Geometry check sheet. Reference: drawing and pictorial views, mm from the part's lowest x, y, z. A direction names the side the tool comes from. Give positions to 0.01 mm unless a question says otherwise; leave off trailing zeros. Order: outer loops, then holes, each group sorted by start corner. A loop starts at its lowest first (then second) coordinate and runs counter-clockwise, first axis right, second up.
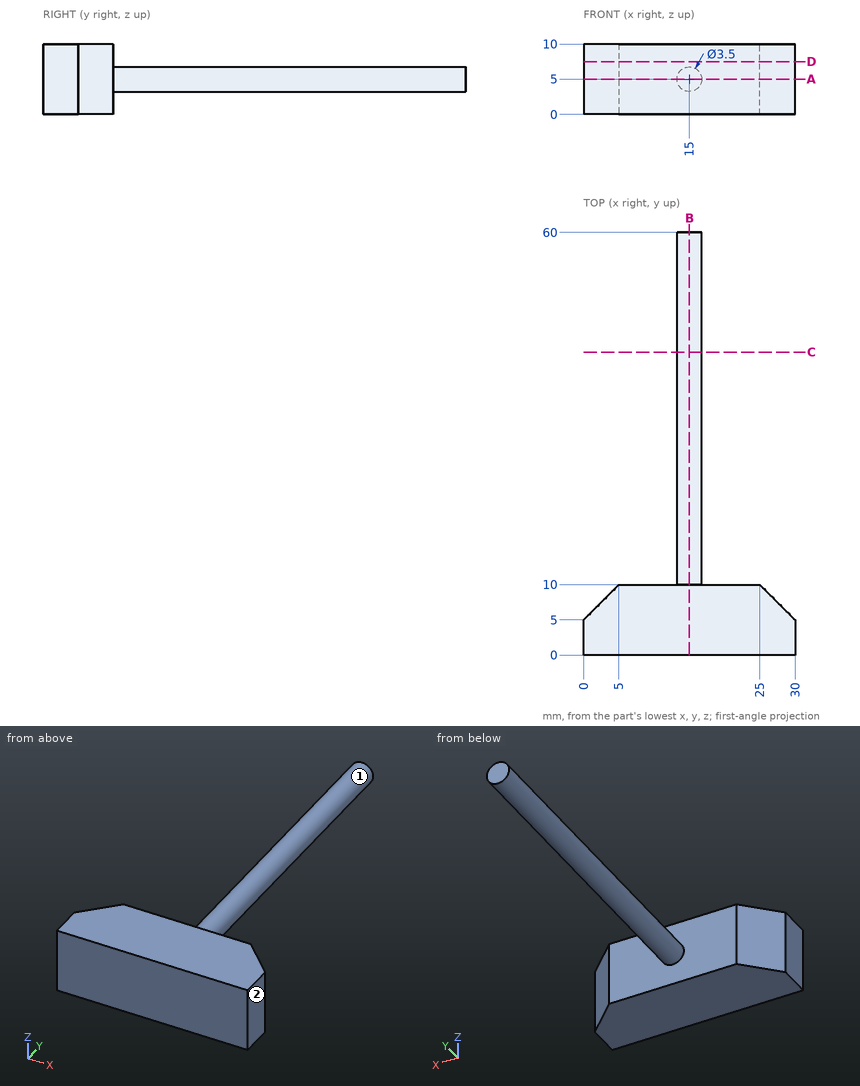
1) Section check B-B, the plane x = 15. Record the cut outline in (y, z), then the cut area to 3 significant figures.
Recorded:
outline: (0, 0) - (10, 0) - (10, 3.25) - (60, 3.25) - (60, 6.75) - (10, 6.75) - (10, 10) - (0, 10) - close
area: 275 mm2
2) Set-up check for the marked faces 1 and 2: record each of +Z, -Z, +X, -X, +Y, -Y from which the full face is reachable in a straight line by a thin tool's end or side.
Recorded:
face 1: +Y
face 2: +Z, -Z, +X, +Y, -Y
3) Section check C-C, the plane y = 43. Record the cut outline in (x, z), then the cut area to 3 significant figures.
Recorded:
outline: circle Ø3.5 at (15, 5)
area: 9.62 mm2
4) Depth check by flat-ended pin: pin 1 Ø1.5 at (x, z) = (21, 3.5) entering from +Y; pin 2 Ø2 at (x, y) = (19.5, 13.5) entering from -Z; pin 3 Ø3 at (x, z) = (16.5, 9) entering from -Y; pin 4 Ø4 at (y, z) = (8, 3.5) entering from +X. Enter the tip coordinate at first touch or a pass-through.
Recorded:
pin 1: stops at y = 10
pin 2: passes through
pin 3: stops at y = 0
pin 4: stops at x = 29
5) Section check D-D, the plane z = 7.5. Record the cut outline in (x, y).
Recorded:
outline: (0, 0) - (30, 0) - (30, 5) - (25, 10) - (5, 10) - (0, 5) - close
6) Section check A-A, the plane z = 5. Record the cut outline in (x, y), then the cut area to 3 significant figures.
Recorded:
outline: (0, 0) - (30, 0) - (30, 5) - (25, 10) - (16.75, 10) - (16.75, 60) - (13.25, 60) - (13.25, 10) - (5, 10) - (0, 5) - close
area: 450 mm2
7) Material ranges on L1, parallel to Y at x = 18.5, z = 4.5; L2, parallel to X at y = 7.5, z = 6.5; L3, parallel to Y at x = 1.75, z = 3.5, recorded low to high.
Recorded:
L1: y = 0 to 10
L2: x = 2.5 to 27.5
L3: y = 0 to 6.75
